The model under review builds one solid part; all positions refer to its coordinate system, in mm. A direction names the side the tool comes from. Round coordinates to 2 decimals unless told otherwise and drop trailing zeros.
Autodesk Inventor part; units mm, degrees
ref_plane "YZ Plane" through (0, 0, 0) normal (1, 0, 0) x (0, 1, 0)
ref_plane "XZ Plane" through (0, 0, 0) normal (0, 1, 0) x (-1, 0, 0)
ref_plane "XY Plane" through (0, 0, 0) normal (0, 0, 1) x (1, 0, 0)
sketch "Sketch1" plane through (0, 0, 0) normal (0, 0, 1) x (1, 0, 0)
  arc A0 (-11.5663, -0.1236) -> (-11.886, 0.8407) centre (-11.7326, 0.3564) ccw
  arc A1 (-11.5663, -0.1236) -> (-10.4403, -2.6494) centre (6.35, 6.35) ccw
  arc A2 (-12.7, 6.35) -> (-11.886, 0.8407) centre (6.35, 6.35) ccw
  arc A3 (-9.9367, -3.5317) -> (-10.4403, -2.6494) centre (-10.1943, -3.0939) ccw
  line L0 (-12.7, 6.35) -> (-12.7, 9.5504)
  arc A4 (-9.9367, -3.5317) -> (-3.5317, -9.9367) centre (6.35, 6.35) ccw
  arc A5 (-12.7, 9.5504) -> (-12.7, 10.5664) centre (-12.7, 10.0584) ccw
  arc A6 (-2.6494, -10.4403) -> (-3.5317, -9.9367) centre (-3.0939, -10.1943) ccw
  line L1 (-12.7, 10.5664) -> (-12.7, 10.5918)
  arc A7 (-2.6494, -10.4403) -> (-0.1348, -11.5623) centre (6.35, 6.35) ccw
  arc A8 (-10.5918, 12.7) -> (-12.7, 10.5918) centre (-10.5918, 10.5918) ccw
  arc A9 (0.8294, -11.8825) -> (-0.1348, -11.5623) centre (0.3459, -11.7266) ccw
  line L2 (-10.5918, 12.7) -> (-10.5664, 12.7)
  arc A10 (0.8294, -11.8825) -> (6.35, -12.7) centre (6.35, 6.35) ccw
  arc A11 (-10.5664, 12.7) -> (-9.5504, 12.7) centre (-10.0584, 12.7) ccw
  line L3 (9.5504, -12.7) -> (6.35, -12.7)
  line L4 (-9.5504, 12.7) -> (-6.3246, 12.7)
  arc A12 (10.5664, -12.7) -> (9.5504, -12.7) centre (10.0584, -12.7) ccw
  arc A13 (-6.3246, 12.7) -> (-5.3086, 12.7) centre (-5.8166, 12.7) ccw
  line L5 (10.5918, -12.7) -> (10.5664, -12.7)
  line L6 (-5.3086, 12.7) -> (-4.3561, 12.7)
  arc A14 (10.5918, -12.7) -> (12.7, -10.5918) centre (10.5918, -10.5918) ccw
  arc A15 (-4.3561, 10.4902) -> (-4.3561, 12.7) centre (-4.3561, 11.5951) ccw
  line L7 (12.7, -10.5664) -> (12.7, -10.5918)
  line L8 (-4.3561, 10.4902) -> (-6.4748, 10.4902)
  arc A16 (12.7, -9.5504) -> (12.7, -10.5664) centre (12.7, -10.0584) ccw
  arc A17 (-6.4748, 10.4902) -> (-7.1932, 8.7558) centre (-6.4748, 9.4742) ccw
  line L9 (12.7, -6.3246) -> (12.7, -9.5504)
  line L10 (-7.1932, 8.7558) -> (-3.8759, 5.4384)
  arc A18 (12.7, -5.3086) -> (12.7, -6.3246) centre (12.7, -5.8166) ccw
  arc A19 (-3.8759, 5.4384) -> (-1.6308, 4.5085) centre (-1.6308, 7.6835) ccw
  line L11 (12.7, -4.3561) -> (12.7, -5.3086)
  line L12 (-1.6308, 4.5085) -> (1.6308, 4.5085)
  arc A20 (12.7, -4.3561) -> (10.4902, -4.3561) centre (11.5951, -4.3561) ccw
  arc A21 (1.6308, 4.5085) -> (3.8759, 5.4384) centre (1.6308, 7.6835) ccw
  line L13 (10.4902, -6.4748) -> (10.4902, -4.3561)
  line L14 (7.1932, 8.7558) -> (3.8759, 5.4384)
  arc A22 (8.7558, -7.1932) -> (10.4902, -6.4748) centre (9.4742, -6.4748) ccw
  arc A23 (7.1932, 8.7558) -> (6.4748, 10.4902) centre (6.4748, 9.4742) ccw
  line L15 (8.7558, -7.1932) -> (5.4384, -3.8759)
  line L16 (6.4748, 10.4902) -> (4.3561, 10.4902)
  arc A24 (4.5085, -1.6308) -> (5.4384, -3.8759) centre (7.6835, -1.6308) ccw
  arc A25 (4.3561, 12.7) -> (4.3561, 10.4902) centre (4.3561, 11.5951) ccw
  line L17 (4.5085, 1.6308) -> (4.5085, -1.6308)
  line L18 (4.3561, 12.7) -> (5.3086, 12.7)
  arc A26 (5.4384, 3.8759) -> (4.5085, 1.6308) centre (7.6835, 1.6308) ccw
  arc A27 (5.3086, 12.7) -> (6.3246, 12.7) centre (5.8166, 12.7) ccw
  line L19 (8.7558, 7.1932) -> (5.4384, 3.8759)
  line L20 (6.3246, 12.7) -> (9.5504, 12.7)
  arc A28 (10.4902, 6.4748) -> (8.7558, 7.1932) centre (9.4742, 6.4748) ccw
  arc A29 (9.5504, 12.7) -> (10.5664, 12.7) centre (10.0584, 12.7) ccw
  line L21 (10.4902, 4.3561) -> (10.4902, 6.4748)
  line L22 (10.5664, 12.7) -> (10.5918, 12.7)
  arc A30 (10.4902, 4.3561) -> (12.7, 4.3561) centre (11.5951, 4.3561) ccw
  arc A31 (12.7, 10.5918) -> (10.5918, 12.7) centre (10.5918, 10.5918) ccw
  line L23 (12.7, 5.3086) -> (12.7, 4.3561)
  line L24 (12.7, 10.5918) -> (12.7, 10.5664)
  arc A32 (12.7, 6.3246) -> (12.7, 5.3086) centre (12.7, 5.8166) ccw
  arc A33 (12.7, 10.5664) -> (12.7, 9.5504) centre (12.7, 10.0584) ccw
  line L25 (12.7, 9.5504) -> (12.7, 6.3246)
  arc A34 (-4.5085, 0.2413) -> (0.2413, -4.5085) centre (0.2413, 0.2413) ccw
  line L26 (0.2413, -4.5085) -> (1.6308, -4.5085)
  line L27 (-4.5085, 1.6308) -> (-4.5085, 0.2413)
  arc A35 (3.8759, -5.4384) -> (1.6308, -4.5085) centre (1.6308, -7.6835) ccw
  arc A36 (-4.5085, 1.6308) -> (-5.4384, 3.8759) centre (-7.6835, 1.6308) ccw
  line L28 (3.8759, -5.4384) -> (7.1927, -8.7553)
  line L29 (-8.7553, 7.1927) -> (-5.4384, 3.8759)
  arc A37 (6.4823, -10.4897) -> (7.1927, -8.7553) centre (6.4743, -9.4737) ccw
  arc A38 (-8.7553, 7.1927) -> (-10.4897, 6.4823) centre (-9.4737, 6.4743) ccw
  arc A39 (-10.4897, 6.4823) -> (6.4823, -10.4897) centre (6.35, 6.35) ccw
  circle A40 centre (0, 0) radius 2.6035
extrude "Extrusion1" add sketch "Sketch1" against normal blind 304.8
properties part number "1012"
(1) To check wall thickness, follow L1, parallel to Y at x = 2, z = -161; L2, parallel to X at y = -1.25, z = -158.5; L3, parallel to X at y = 1.75, z = -139. State the ranges of each line that lie inside material, in increasing order.
(2) The part is to be moulded in two halves that separate along Y. For faces 3 (the flat face through (3, 0, 0)), 4 (the cylindrical face through (-3.154, -3.08, -150.266)), 5 (the cylindrical face through (-12.5, 3.6, -150.3)), say which applies: pulls with the +Y half, pulls with the -Y half, needs draft (parallel to the pull), parting line crosses it, or undercut.
(3) Clearance check with flat-ended pins moving along their axes: P1, Ø4, axis at y = 1, z = -129.5, coming from the -X side; P2, Ø0.6, axis at x = 5.5, z = -84, coming from the -Y side; P3, Ø1, axis at x = 0.5, z = -220, coming from the +Y side; P4, Ø8, axis at x = -7, y = 9, coming from the +Z side. State where each tip first meets the part, or that it passes through.
(4) Tool access review of faces 1 (the flat face through (3, 0, -304.8)), 2 (the cylindrical face through (-5.689, -5.425, -150.266)): name each direction out of +Z, -Z, +X, -X, +Y, -Y from which nothing blocks a thin tool from reaching the whole face with its end or side.
(5) We need section A-A (z = -94.5). Count the separate pieces of the cut face and the enclosed holes in it, and give its area (3 significant figures).
Verdict:
1. L1: y = -12.2 to -9.92, -4.53 to -1.67, 1.67 to 4.53
1. L2: x = -11.12 to -8.68, -4.27 to -2.28, 2.28 to 4.51
1. L3: x = -12.14 to -9.85, -4.51 to -1.93, 1.93 to 4.51
2. face 3: needs draft
2. face 4: undercut
2. face 5: pulls with the -Y half
3. P1: stops at x = -12.4
3. P2: stops at y = -12.69
3. P3: stops at y = 4.51
3. P4: stops at z = 0
4. face 1: -Z, +X, -X, +Y, -Y
4. face 2: +Z, -Z
5. separate pieces: 1
5. enclosed holes: 2
5. area: 269 mm2
